Check sheet for the modelled part. Datum: model origin and axes. Units: mm. A direction names the side the tool comes from. Give positions to 0.01 mm unless a question says otherwise; leave off trailing zeros. Write each loop counter-clockwise with the first axis right and the second up, starting at its lowest first coordinate (ties: lowest second). Pieces come first, ordered by that corner, then holes. Notation, with made-up numbers: M 63.25,-8 L 77.25,-8 A30 cw 77.25,15 Z; hole C -9,82.25 d2. An arc over 180 degrees is marked long. One line per item, written item: value. Start each with the question number.
from build123d import *

# Parameters (mm, degrees)
SKETCH1_R           = 8
BOSS_EXTRUDE1_DEPTH = 3.5
SKETCH2_R           = 6
BOSS_EXTRUDE2_DEPTH = 5
SKETCH3_R           = 8
BOSS_EXTRUDE3_DEPTH = 3
SKETCH4_R           = 4.5
BOSS_EXTRUDE4_DEPTH = 6
SKETCH5_R           = 12.5
BOSS_EXTRUDE5_DEPTH = 32
SKETCH6_R           = 3
BOSS_EXTRUDE6_DEPTH = 3
SKETCH7_W           = 16
SKETCH7_H           = 16
BOSS_EXTRUDE7_DEPTH = 11
SKETCH8_R           = 4
BOSS_EXTRUDE8_DEPTH = 3
SKETCH10_R          = 1.5
CUT_EXTRUDE1_DEPTH  = 2


with BuildPart() as part:
    # Sketch1 → Boss-Extrude1 (new body)
    with BuildSketch(Plane.XY):
        Circle(SKETCH1_R)
    extrude(amount=BOSS_EXTRUDE1_DEPTH)

    # Sketch2 → Boss-Extrude2 (add)
    with BuildSketch(Plane.XY.offset(3.5)):
        Circle(SKETCH2_R)
    extrude(amount=BOSS_EXTRUDE2_DEPTH)

    # Sketch3 → Boss-Extrude3 (add)
    with BuildSketch(Plane.XY.offset(8.5)):
        Circle(SKETCH3_R)
    extrude(amount=BOSS_EXTRUDE3_DEPTH)

    # Sketch4 → Boss-Extrude4 (add)
    with BuildSketch(Plane.XY.offset(11.5)):
        Circle(SKETCH4_R)
    extrude(amount=BOSS_EXTRUDE4_DEPTH)

    # Sketch5 → Boss-Extrude5 (add)
    with BuildSketch(Plane.XY.offset(17.5)):
        Circle(SKETCH5_R)
    extrude(amount=BOSS_EXTRUDE5_DEPTH)

    # Sketch6 → Boss-Extrude6 (add)
    with BuildSketch(Plane.XY.offset(49.5)):
        Circle(SKETCH6_R)
    extrude(amount=BOSS_EXTRUDE6_DEPTH)

    # Sketch7 → Boss-Extrude7 (add)
    with BuildSketch(Plane.XY.offset(52.5)):
        with Locations((4, 0)):
            Rectangle(SKETCH7_W, SKETCH7_H)
    extrude(amount=BOSS_EXTRUDE7_DEPTH)

    # Sketch8 → Boss-Extrude8 (add)
    with BuildSketch(Plane.XY.offset(63.5)):
        with Locations(Location((0, 0, 0), (0, 0, 180))):
            Circle(SKETCH8_R)
    extrude(amount=BOSS_EXTRUDE8_DEPTH)

    # Sketch10 → Cut-Extrude1 (cut)
    with BuildSketch(Plane(origin=(0, 0, 0), x_dir=(-1, 0, 0), z_dir=(0, 0, -1))):
        Circle(SKETCH10_R)
    extrude(amount=-CUT_EXTRUDE1_DEPTH, mode=Mode.SUBTRACT)

    # Loft1: read off the stored shape, not the designer's step
    # Loft1: loft between two sections, ruled curve by curve
    loft1_from = [
        Edge.make_bspline([(-0.247162936, 0.037556397, 68.5), (-0.172050142, 0.53188227, 68.5), (0.322275731, 0.456769475, 68.5), (0.247162936, -0.037556397, 68.5), (0.172050142, -0.53188227, 68.5), (-0.322275731, -0.456769475, 68.5), (-0.247162936, 0.037556397, 68.5)], [0, 0, 0, 0, 0.5, 0.5, 0.5, 1, 1, 1, 1], 3, [1, 0.333333333, 0.333333333, 1, 0.333333333, 0.333333333, 1]),
    ]
    loft1_to = [
        Edge.make_bspline([(-1.919178945, -0.562807407, 66.5), (-3.044793759, 3.275550482, 66.5), (0.79356413, 4.401165297, 66.5), (1.919178945, 0.562807407, 66.5), (3.044793759, -3.275550482, 66.5), (-0.79356413, -4.401165297, 66.5), (-1.919178945, -0.562807407, 66.5)], [0, 0, 0, 0, 0.5, 0.5, 0.5, 1, 1, 1, 1], 3, [1, 0.333333333, 0.333333333, 1, 0.333333333, 0.333333333, 1]),
    ]
    loft1 = Solid(Shell([*[Face.make_surface_from_curves(loft1_from[k], loft1_to[k]) for k in range(1)], Face(Wire(loft1_from)), Face(Wire(loft1_to))]))
    add(loft1)


solid = part.part
1) Tool access check on faces 4 (the cylindrical face through (11.923, 3.755, 33.276)), 5 (the flat face through (4, -8, 58)), 6 (the flat face through (12, 0, 58)), 7 (the cylindrical face through (-6, 0, 6)), 8 (the flat face through (-1, 2, 66.5)). Record the directions out of +Z, -Z, +X, -X, +Y, -Y that give a thin tool (end or side, any length) a straight path to the whole face; none if there is none.
2) Cross-section at B-B (y = -7). Record the boundary of the cut face in (x, z), plus the area to 3 significant figures.
3) Material ranges on L1, parallel to Z at x = 1.75, y = 4.5; L2, parallel to Y at x = 0, z = 0.95; L3, parallel to Z at x = -4.25, y = 4, recorded low to high. Write a range as from..to.
4) Cross-section at A-A (x = 9.5). Record the boundary of the cut face in (y, z), plus the area to 3 significant figures.
5) Draft check along Z on faces 1 (the flat face through (4, 8, 58)), 2 (the flat face through (6, 0, 63.5)), 3 (the flat face through (3.4, -3.4, 11.5)). Enter one of: released by +Z, released by -Z, zero draft, split by the parting line, or undercut.
6) Cross-section at D-D (z = 62.5). Record the boundary of the cut face in (x, y), plus the area to 3 significant figures.
7) Cross-section at C-C (z = 12.5). Record the boundary of the cut face in (x, y), plus the area to 3 significant figures.
8) Gauge pin test, flat ends, axial feed: pin 1 (8 mm diameter, centred on x = -3.5, y = -5.5, fed in from +Z); pin 2 (1.5 mm diameter, centred on x = -0.5, y = 0.5, fed in from -Z); pin 3 (3 mm diameter, centred on x = 2, z = 47.5, fed in from +Y). Record the tip position at first contact, or that the pin passes through.
Data:
1. face 4: -Z
1. face 5: +Z, +X, -X, -Y
1. face 6: +Z, +X, +Y, -Y
1. face 7: none
1. face 8: +Z
2. outline: M -10.36,17.5 L 10.36,17.5 L 10.36,49.5 L -10.36,49.5 Z; M -4,52.5 L 12,52.5 L 12,63.5 L -4,63.5 Z; M -3.87,0 L 3.87,0 L 3.87,3.5 L -3.87,3.5 Z; M -3.87,8.5 L 3.87,8.5 L 3.87,11.5 L -3.87,11.5 Z
2. area: 889 mm2
3. L1: z = 0..11.5, 17.5..49.5, 52.5..63.5
3. L2: y = -8..-1.5, 1.5..8
3. L3: z = 0..11.5, 17.5..49.5
4. outline: M -8.12,17.5 L 8.12,17.5 L 8.12,49.5 L -8.12,49.5 Z; M -8,52.5 L 8,52.5 L 8,63.5 L -8,63.5 Z
4. area: 696 mm2
5. face 1: zero draft
5. face 2: released by +Z
5. face 3: undercut
6. outline: M -4,-8 L 12,-8 L 12,8 L -4,8 Z
6. area: 256 mm2
7. outline: C 0,0 d9
7. area: 63.6 mm2
8. pin 1: stops at z = 66.5
8. pin 2: stops at z = 2
8. pin 3: stops at y = 12.49
